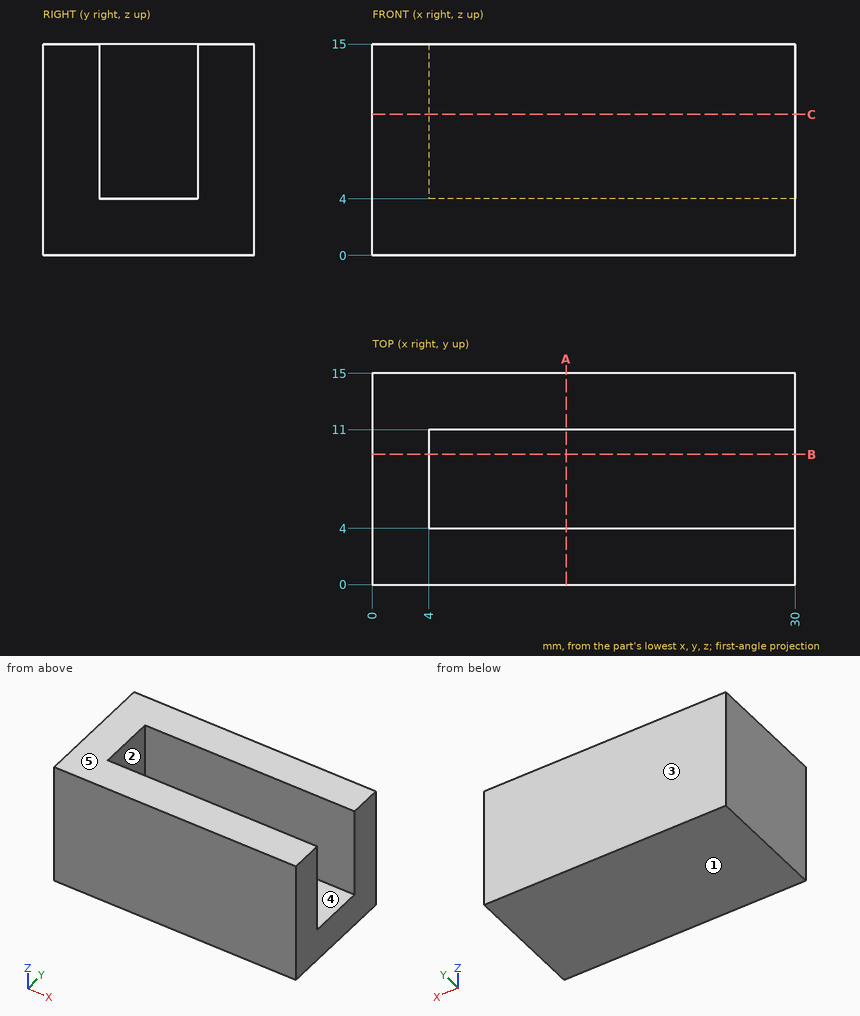
Geometry check sheet. Reference: drawing and pictorial views, mm from the part's lowest x, y, z. A direction names the side the tool comes from. Give positions to 0.01 mm unless a question says otherwise; leave off trailing zeros. Loops run counter-clockwise (first coordinate to the right, second up) from the corner with the lowest first, then second, coordinate; pieces in that order, holes last.
1. Thickness scan on line 1 (Y direction, x = 22.5, z = 12); line 2 (X direction, y = 9.75, z = 12.75). Record the ranges inside material, lowest first.
2. Go/stop test with flat-tipped pins: pin 1 Ø3 at (x, y) = (12.5, 2) entering from -Z; pin 2 Ø1 at (x, y) = (22.5, 5) entering from +Z. Record where each tip stops, or that it passes through.
3. Section check B-B, the plane y = 9.25. Enter the section's corners in (x, z).
4. Section check A-A, the plane x = 13.75. Enter the section's corners in (y, z), then the cut area to 3 significant figures.
5. Section check C-C, the plane z = 10. Enter the section's corners in (x, y), then the cut area to 3 significant figures.
6. Mould release check, pull along Y, two halves, no side actions. Record for the marked faces 3, 4 and 5: released by +Y, released by -Y, zero draft, split by the parting line, or undercut.
7. Set-up check for the marked faces 1 and 2: record each of +Z, -Z, +X, -X, +Y, -Y from which the full face is reachable in a straight line by a thin tool's end or side.
Geometry says:
1. line 1: y = 0 to 4, 11 to 15
1. line 2: x = 0 to 4
2. pin 1: stops at z = 0
2. pin 2: stops at z = 4
3. outline: (0, 0) - (30, 0) - (30, 4) - (4, 4) - (4, 15) - (0, 15) - close
4. outline: (0, 0) - (15, 0) - (15, 15) - (11, 15) - (11, 4) - (4, 4) - (4, 15) - (0, 15) - close
4. area: 148 mm2
5. outline: (0, 0) - (30, 0) - (30, 4) - (4, 4) - (4, 11) - (30, 11) - (30, 15) - (0, 15) - close
5. area: 268 mm2
6. face 3: released by +Y
6. face 4: undercut
6. face 5: zero draft
7. face 1: -Z, +X, -X, +Y, -Y
7. face 2: +Z, +X
